from build123d import *

# Parameters (mm, degrees)
F0_R       = 49.5
F0_R_2     = 38.5
F1_DEPTH   = 70
F2_R       = 54.3323959341
F2_R_2     = 47.75
F3_DEPTH   = 1.75
F6_R       = 54.3323959341
F6_R_2     = 47.75
F8_DEPTH   = 1.75
F7_R       = 54.3323959341
F7_R_2     = 47.75
F9_DEPTH   = 1.75
F10_W      = 0.1
F10_H      = 63.4597092867
F12_DEPTH  = 75
F12_FACE_W = 63.4597092867
F12_FACE_H = 150
F13_ANGLE  = 240
F14_DEPTH  = 150


with BuildPart() as f1:
    # F0 (on Top) → F1 (new body, symmetric)
    with BuildSketch(Plane.XY):
        Circle(F0_R)
        Circle(F0_R_2, mode=Mode.SUBTRACT)
    extrude(amount=F1_DEPTH, both=True)

    # F2 (on Top) → F3 (cut, symmetric)
    with BuildSketch(Plane.XY):
        Circle(F2_R)
        Circle(F2_R_2, mode=Mode.SUBTRACT)
    extrude(amount=F3_DEPTH, both=True, mode=Mode.SUBTRACT)

    # F6 (on offset) → F8 (cut, symmetric)
    with BuildSketch(Plane.XY.offset(46)):
        Circle(F6_R)
        Circle(F6_R_2, mode=Mode.SUBTRACT)
    extrude(amount=F8_DEPTH, both=True, mode=Mode.SUBTRACT)

    # F7 (on offset) → F9 (cut, symmetric)
    with BuildSketch(Plane.XY.offset(-46)):
        Circle(F7_R)
        Circle(F7_R_2, mode=Mode.SUBTRACT)
    extrude(amount=F9_DEPTH, both=True, mode=Mode.SUBTRACT)

    # F10 (on Top) → F12 (join, symmetric)
    with BuildSketch(Plane.XY):
        with Locations((0.05, 31.7298546433)):
            Rectangle(F10_W, F10_H)
    extrude(amount=F12_DEPTH, both=True)


with BuildPart() as f13:
    # F12_face (on face) → F13 (revolve)
    with BuildSketch(Plane(origin=(0, 29.4058824781, 0), x_dir=(0, -1, 0), z_dir=(-1, 0, 0))):
        with Locations((-2.3239721652, 0)):
            Rectangle(F12_FACE_W, F12_FACE_H)
        Polygon((-9.0941175219, -70), (-20.0941175219, -70), (-20.0941175219, -47.75), (-18.3441175219, -47.75), (-18.3441175219, -44.25), (-20.0941175219, -44.25), (-20.0941175219, -1.75), (-18.3441175219, -1.75), (-18.3441175219, 1.75), (-20.0941175219, 1.75), (-20.0941175219, 44.25), (-18.3441175219, 44.25), (-18.3441175219, 47.75), (-20.0941175219, 47.75), (-20.0941175219, 70), (-9.0941175219, 70), align=None, mode=Mode.SUBTRACT)
    revolve(axis=Axis((0, 0, -0.0270418823), (0, 0, 1)), revolution_arc=F13_ANGLE)


with BuildPart() as f14_tool:
    # F14 (cut): a face of the model
    f14_faces = [f13.part.faces().sort_by_distance(p)[0] for p in [
        (-15.1498896302, -8.7467928562, 75),
    ]]
    extrude(f14_faces, amount=-F14_DEPTH)


with BuildPart() as f1_1:
    add(f1.part)

    # F14: cut by f14_tool
    add(f14_tool.part, mode=Mode.SUBTRACT)


with BuildPart() as f13_1:
    add(f13.part)

    # F14: cut by f14_tool
    add(f14_tool.part, mode=Mode.SUBTRACT)


solid = f1_1.part
The model under review builds one solid part; all positions refer to its coordinate system, in mm. A direction names the side the tool comes from. Round coordinates to 2 decimals unless told otherwise and drop trailing zeros. Order: outer loops, then holes, each group sorted by start corner. A loop starts at its lowest first (then second) coordinate and runs counter-clockwise, first axis right, second up. Notation, with made-up numbers: (-26, -20) -> (13, -20) arc R16 ccw to (13, -2) -> close; hole circle Ø11 at (54.25, 84). An arc over 180 degrees is marked (long way). Write item = value, one per line. Start each with the question number.
Item 1: Mouldability with a two-part tool opening along Z and no side actions: class faces 1 (the face through (43.25, 24.08, 59.03)), 2 (the face through (41, 26, 1.75)), 3 (the face through (36, 18, -70)) as released by +Z, released by -Z, zero draft, split by the parting line, or undercut.
Item 2: Consider section D-D on x = 18.5. Write out the cut boundary in (y, z), plus the area to 3 significant figures.
Item 3: Consider section A-A on z = -61. Write out the cut boundary in (x, y).
Item 4: For faces 4 (the face through (36, 18, 70)), 5 (the face through (41.722, 23.223, -0.024)), 6 (the face through (33.645, 18.716, -0.98)), list the 3-axis set-ups (+Z, -Z, +X, -X, +Y, -Y) from which the entire face can be reached by the end or side of a thin tool; tool diameter is ignored.
Item 5: For line 1 along Z through (x, y) = (36.5, 14); line 2 along Y through (x, z) = (34, -33); line 3 along X through (y, z) = (-11.5, 22), list the stretches that pass through material, from the lowest coordinate up.
Item 6: Consider section C-C on x = 36. Write out the cut boundary in (y, z), plus the area to 3 significant figures.
Item 7: Clearance check with flat-ended pins moving along their axes: pin 1 Ø24.5 at (x, y) = (29, 27) entering from +Z; pin 2 Ø8 at (y, z) = (39, -13) entering from +X; pin 3 Ø19 at (y, z) = (44, 15) entering from +X; pin 4 Ø5 at (y, z) = (41, 28) entering from -X. State where each tip first meets the part, or that it passes through.
Item 8: Consider section B-B on y = 27. Write out the cut boundary in (x, z), plus the area to 3 significant figures.
Conclusion:
q1.face_1 = zero draft
q1.face_2 = undercut
q1.face_3 = released by -Z
q2.outline = (33.76, -70) -> (45.91, -70) -> (45.91, -47.75) -> (44.02, -47.75) -> (44.02, -44.25) -> (45.91, -44.25) -> (45.91, -1.75) -> (44.02, -1.75) -> (44.02, 1.75) -> (45.91, 1.75) -> (45.91, 44.25) -> (44.02, 44.25) -> (44.02, 47.75) -> (45.91, 47.75) -> (45.91, 70) -> (33.76, 70) -> close
q2.area = 1,680 mm2
q3.outline = (0, 0) -> (0.1, 0) -> (0.1, 38.5) arc R38.5 cw to (33.34, -19.25) -> (42.87, -24.75) arc R49.5 ccw to (0.1, 49.5) -> (0.1, 63.46) -> (0, 63.46) -> close
q4.face_4 = +Z, +X, +Y, -Y
q4.face_5 = +X
q4.face_6 = +Z, -Z
q5.line_1 = -70 to 70
q5.line_2 = -19.63 to -18.06, 18.06 to 35.98
q5.line_3 = 36.74 to 48.15
q6.outline = (-20.78, -70) -> (-13.65, -70) -> (-13.65, 70) -> (-20.78, 70) -> close; (13.65, -70) -> (33.97, -70) -> (33.97, -47.75) -> (31.37, -47.75) -> (31.37, -44.25) -> (33.97, -44.25) -> (33.97, -1.75) -> (31.37, -1.75) -> (31.37, 1.75) -> (33.97, 1.75) -> (33.97, 44.25) -> (31.37, 44.25) -> (31.37, 47.75) -> (33.97, 47.75) -> (33.97, 70) -> (13.65, 70) -> close
q6.area = 3,820 mm2
q7.pin_1 = 70
q7.pin_2 = 35
q7.pin_3 = 35.5
q7.pin_4 = 0
q8.outline = (0, -75) -> (0.1, -75) -> (0.1, 75) -> (0, 75) -> close; (27.45, -70) -> (41.49, -70) -> (41.49, -47.75) -> (39.38, -47.75) -> (39.38, -44.25) -> (41.49, -44.25) -> (41.49, -1.75) -> (39.38, -1.75) -> (39.38, 1.75) -> (41.49, 1.75) -> (41.49, 44.25) -> (39.38, 44.25) -> (39.38, 47.75) -> (41.49, 47.75) -> (41.49, 70) -> (27.45, 70) -> close
q8.area = 1,960 mm2
